Build history of the part. All positions in model axes, mm. Face numbers are marked on the shaded views. A direction names the side the tool comes from. Give positions to 0.01 mm unless a question says otherwise; leave off trailing zeros. Order: outer loops, then holes, each group sorted by start corner. A loop starts at its lowest first (then second) coordinate and runs counter-clockwise, first axis right, second up. Notation, with made-up numbers: (37.5, 67.5) - (44.5, 67.5) arc R30 ccw to (44.5, 104.5) - close; hole circle Ø2 at (66, 67.25). An arc over 180 degrees is marked (long way). Use a Markdown table: item, result. Add a question column.
(1) Slice it at C-C (z = -31). Write the cut outline in (x, y).
(2) Flat gauge pins, fed straight in: pin 1 (9.5 mm diameter, centred on x = 136, y = -14, fed in from -Z); pin 2 (11.5 mm diameter, centred on x = -51, y = -127, fed in from +Z); pin 3 (10 mm diameter, centred on y = -82, z = 22.5, fed in from +X). Where does each tip first touch, or does it go through?
(3) Slice it at A-A (x = 0). Count the separate pieces of the cut face and the enclosed holes in it, then the cut area to 3 significant figures.
(4) Wall check: line 1 (Y direction, x = 0, z = 38); line 2 (X direction, y = 94, z = 11); line 3 (X direction, y = 53, z = 17). Give the ranges that are in metal, low to high.
(5) Mould opens along Y. For the marked faces 3 and 4 say: +Y half, -Y half, draft (parallel to the pull), parting line (faces both ways), or undercut.
(6) Which spindle directions (+Z, -Z, +X, -X, +Y, -Y) get a long thin tool onto all of the face, cutting with end or side? Do the marked faces 1 and 2. Say none if no direction does.
from build123d import *

# Parameters (mm, degrees)
CUT_EXTRUDE1_DEPTH      = 246.560583156
CUT_EXTRUDE1_DEPTH_BACK = 246.560583156


with BuildPart() as part:
    # Sketch2 → Revolve1 (revolve)
    with BuildSketch(Plane(origin=(0, 0, 0), x_dir=(1, 0, 0), z_dir=(0, 1, 0))):
        with BuildLine():
            Line((-47.5, -40), (-114, -40))
            ThreePointArc((-114, -40), (-123.899494937, -35.899494937), (-128, -26))
            Line((-128, -26), (-130, -26))
            ThreePointArc((-130, -26), (-130.749756335, -18.015609771), (-131, -10))
            Line((-131, -10), (-151, -10))
            ThreePointArc((-151, -10), (-157.444175053, -16.906401533), (-160, -26))
            Line((-160, -26), (-170, -26))
            Line((-170, -26), (-170, -24))
            Line((-170, -24), (-164, -24))
            ThreePointArc((-164, -24), (-158.990908339, 0), (-164, 24))
            Line((-164, 24), (-170, 24))
            Line((-170, 24), (-170, 26))
            Line((-170, 26), (-160, 26))
            ThreePointArc((-160, 26), (-157.444175053, 16.906401533), (-151, 10))
            Line((-151, 10), (-131, 10))
            ThreePointArc((-131, 10), (-130.749756335, 18.015609771), (-130, 26))
            Line((-130, 26), (-128, 26))
            ThreePointArc((-128, 26), (-123.899494937, 35.899494937), (-114, 40))
            Line((-114, 40), (-47.5, 40))
            Line((-47.5, 40), (-47.5, 37))
            Line((-47.5, 37), (-30, 37))
            Line((-30, 37), (-30, -37))
            Line((-30, -37), (-47.5, -37))
            Line((-47.5, -37), (-47.5, -40))
        make_face()
    revolve(axis=Axis((0, 0, -135.367425902), (0, 0, 1)))

    # Sketch3 → Cut-Extrude1 (cut, two sides: drawn at the far end of the back side and taken through both)
    with BuildSketch(Plane.XY.offset(10).offset(-CUT_EXTRUDE1_DEPTH_BACK)):
        with BuildLine():
            ThreePointArc((-16.775359417, 141.517465908), (-17.663637735, 146.86526576), (-22.5, 149.314265896))
            ThreePointArc((-22.5, 149.314265896), (-65.516444607, 136.046299053), (-102.710073317, 110.687130414))
            ThreePointArc((-102.710073317, 110.687130414), (-103.810790461, 105.378983525), (-100.183544647, 101.350200901))
            Line((-100.183544647, 101.350200901), (-91.789558594, 98.103510563))
            ThreePointArc((-91.789558594, 98.103510563), (-89.333916802, 97.632512022), (-86.869399468, 98.054614557))
            ThreePointArc((-86.869399468, 98.054614557), (-56.838769824, 118.026921695), (-22.5, 129.053283569))
            ThreePointArc((-22.5, 129.053283569), (-20.633385525, 130.716944184), (-19.470559398, 132.930505034))
            Line((-19.470559398, 132.930505034), (-16.775359417, 141.517465908))
        make_face()
        with BuildLine():
            Line((-97.575757874, 87.406930362), (-113.234667829, 99.894494351))
            ThreePointArc((-113.234667829, 99.894494351), (-118.056553853, 94.146960081), (-122.587014857, 88.167022114))
            Line((-122.587014857, 88.167022114), (-106.928104902, 75.679458125))
            ThreePointArc((-106.928104902, 75.679458125), (-102.419924203, 81.677164043), (-97.575757874, 87.406930362))
        make_face()
        with BuildLine():
            ThreePointArc((-121.102075685, 75.119192657), (-125.836986444, 77.759007373), (-130.767114401, 75.504713703))
            ThreePointArc((-130.767114401, 75.504713703), (-147.214114739, 33.600661027), (-150.577366523, -11.289671876))
            ThreePointArc((-150.577366523, -11.289671876), (-147.113576085, -15.459822645), (-141.70219622, -15.135832553))
            Line((-141.70219622, -15.135832553), (-133.9302668, -10.597428308))
            ThreePointArc((-133.9302668, -10.597428308), (-132.030957698, -8.971193032), (-130.824369324, -6.781179166))
            ThreePointArc((-130.824369324, -6.781179166), (-127.715556496, 29.150242348), (-114.926440552, 62.872197846))
            ThreePointArc((-114.926440552, 62.872197846), (-115.063327708, 65.368851235), (-116.068949037, 67.658117926))
            Line((-116.068949037, 67.658117926), (-121.102075685, 75.119192657))
        make_face()
        with BuildLine():
            Line((-129.174979886, -21.790469739), (-148.701321217, -26.247229726))
            ThreePointArc((-148.701321217, -26.247229726), (-147.214114739, -33.600661027), (-145.363507208, -40.871148409))
            Line((-145.363507208, -40.871148409), (-125.837165877, -36.414388422))
            ThreePointArc((-125.837165877, -36.414388422), (-127.715556496, -29.150242348), (-129.174979886, -21.790469739))
        make_face()
        with BuildLine():
            ThreePointArc((-134.23645893, -47.845364818), (-139.252517754, -49.901369561), (-140.563924495, -55.161427924))
            ThreePointArc((-140.563924495, -55.161427924), (-118.056553853, -94.146960081), (-85.056831518, -124.765120976))
            ThreePointArc((-85.056831518, -124.765120976), (-79.636838347, -124.65706704), (-76.516203841, -120.224275379))
            Line((-76.516203841, -120.224275379), (-75.218752425, -111.318287515))
            ThreePointArc((-75.218752425, -111.318287515), (-75.305994506, -108.819406755), (-76.265920748, -106.510606666))
            ThreePointArc((-76.265920748, -106.510606666), (-102.419924203, -81.677164043), (-120.810927296, -50.652935214))
            ThreePointArc((-120.810927296, -50.652935214), (-122.848237262, -49.203319975), (-125.265052676, -48.562211955))
            Line((-125.265052676, -48.562211955), (-134.23645893, -47.845364818))
        make_face()
        with BuildLine():
            Line((-63.502807355, -114.579201682), (-72.192846774, -132.624254474))
            ThreePointArc((-72.192846774, -132.624254474), (-65.516444607, -136.046299053), (-58.678313755, -139.13251056))
            Line((-58.678313755, -139.13251056), (-49.988274336, -121.087457769))
            ThreePointArc((-49.988274336, -121.087457769), (-56.838769824, -118.026921695), (-63.502807355, -114.579201682))
        make_face()
        with BuildLine():
            ThreePointArc((-46.288050676, -134.781386717), (-47.808062962, -139.984997413), (-44.513232463, -144.289889236))
            ThreePointArc((-44.513232463, -144.289889236), (0, -151), (44.513232463, -144.289889236))
            ThreePointArc((44.513232463, -144.289889236), (47.808062962, -139.984997413), (46.288050676, -134.781386717))
            Line((46.288050676, -134.781386717), (40.134016708, -128.214205744))
            ThreePointArc((40.134016708, -128.214205744), (38.125918511, -126.724387679), (35.722321693, -126.035374927))
            ThreePointArc((35.722321693, -126.035374927), (0, -131), (-35.722321693, -126.035374927))
            ThreePointArc((-35.722321693, -126.035374927), (-38.125918511, -126.724387679), (-40.134016708, -128.214205744))
            Line((-40.134016708, -128.214205744), (-46.288050676, -134.781386717))
        make_face()
        with BuildLine():
            ThreePointArc((85.056831518, -124.765120976), (118.056553853, -94.146960081), (140.563924495, -55.161427924))
            ThreePointArc((140.563924495, -55.161427924), (139.252517754, -49.901369561), (134.23645893, -47.845364818))
            Line((134.23645893, -47.845364818), (125.265052676, -48.562211955))
            ThreePointArc((125.265052676, -48.562211955), (122.848237262, -49.203319975), (120.810927296, -50.652935214))
            ThreePointArc((120.810927296, -50.652935214), (102.419924203, -81.677164043), (76.265920748, -106.510606666))
            ThreePointArc((76.265920748, -106.510606666), (75.305994506, -108.819406755), (75.218752425, -111.318287515))
            Line((75.218752425, -111.318287515), (76.516203841, -120.224275379))
            ThreePointArc((76.516203841, -120.224275379), (79.636838347, -124.65706704), (85.056831518, -124.765120976))
        make_face()
        with BuildLine():
            ThreePointArc((145.363507208, -40.871148409), (147.214114739, -33.600661027), (148.701321217, -26.247229726))
            Line((148.701321217, -26.247229726), (129.174979886, -21.790469739))
            ThreePointArc((129.174979886, -21.790469739), (127.715556496, -29.150242348), (125.837165877, -36.414388422))
            Line((125.837165877, -36.414388422), (145.363507208, -40.871148409))
        make_face()
        with BuildLine():
            ThreePointArc((151, 0), (145.854095374, 39.084304557), (130.767114401, 75.504713703))
            ThreePointArc((130.767114401, 75.504713703), (125.836986444, 77.759007373), (121.102075685, 75.119192657))
            Line((121.102075685, 75.119192657), (116.068949037, 67.658117926))
            ThreePointArc((116.068949037, 67.658117926), (115.063327708, 65.368851235), (114.926440552, 62.872197846))
            ThreePointArc((114.926440552, 62.872197846), (126.918012339, 32.447159257), (131, 0))
            ThreePointArc((131, 0), (130.95608497, -3.391726589), (130.824369324, -6.781179166))
            ThreePointArc((130.824369324, -6.781179166), (132.030957698, -8.971193032), (133.9302668, -10.597428308))
            Line((133.9302668, -10.597428308), (141.70219622, -15.135832553))
            ThreePointArc((141.70219622, -15.135832553), (147.113576085, -15.459822645), (150.577366523, -11.289671876))
            ThreePointArc((150.577366523, -11.289671876), (150.894304639, -5.648789917), (151, 0))
        make_face()
        with BuildLine():
            ThreePointArc((122.587014857, 88.167022114), (118.056553853, 94.146960081), (113.234667829, 99.894494351))
            Line((113.234667829, 99.894494351), (97.575757874, 87.406930362))
            ThreePointArc((97.575757874, 87.406930362), (102.419924203, 81.677164043), (106.928104902, 75.679458125))
            Line((106.928104902, 75.679458125), (122.587014857, 88.167022114))
        make_face()
        with BuildLine():
            ThreePointArc((102.710073317, 110.687130414), (65.516444607, 136.046299053), (22.5, 149.314265896))
            ThreePointArc((22.5, 149.314265896), (17.663637735, 146.86526576), (16.775359417, 141.517465908))
            Line((16.775359417, 141.517465908), (19.470559398, 132.930505034))
            ThreePointArc((19.470559398, 132.930505034), (20.633385525, 130.716944184), (22.5, 129.053283569))
            ThreePointArc((22.5, 129.053283569), (56.838769824, 118.026921695), (86.869399468, 98.054614557))
            ThreePointArc((86.869399468, 98.054614557), (89.333916802, 97.632512022), (91.789558594, 98.103510563))
            Line((91.789558594, 98.103510563), (100.183544647, 101.350200901))
            ThreePointArc((100.183544647, 101.350200901), (103.810790461, 105.378983525), (102.710073317, 110.687130414))
        make_face()
        with BuildLine():
            ThreePointArc((7.5, 150.813626705), (0, 151), (-7.5, 150.813626705))
            Line((-7.5, 150.813626705), (-7.5, 130.785129124))
            ThreePointArc((-7.5, 130.785129124), (0, 131), (7.5, 130.785129124))
            Line((7.5, 130.785129124), (7.5, 150.813626705))
        make_face()
        with BuildLine():
            ThreePointArc((58.678313755, -139.13251056), (65.516444607, -136.046299053), (72.192846774, -132.624254474))
            Line((72.192846774, -132.624254474), (63.502807355, -114.579201682))
            ThreePointArc((63.502807355, -114.579201682), (56.838769824, -118.026921695), (49.988274336, -121.087457769))
            Line((49.988274336, -121.087457769), (58.678313755, -139.13251056))
        make_face()
    extrude(amount=CUT_EXTRUDE1_DEPTH + CUT_EXTRUDE1_DEPTH_BACK, mode=Mode.SUBTRACT)


solid = part.part
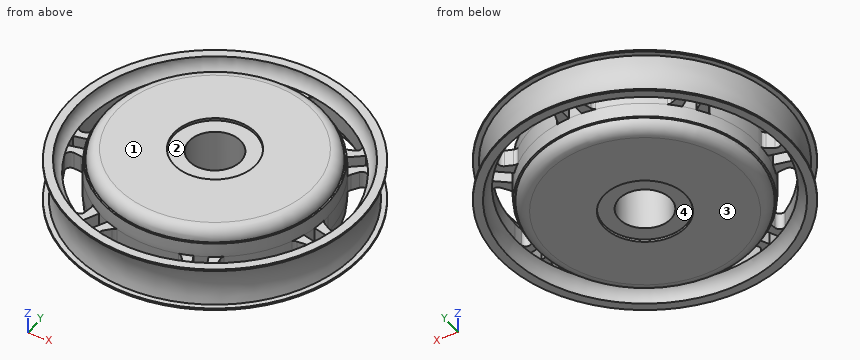
Solution:
| question | item | result |
|---|---|---|
| 1 | outline | circle Ø254.15 at (0, 0); hole circle Ø60 at (0, 0) |
| 2 | pin 1 | z = -10 |
| 2 | pin 2 | z = 10 |
| 2 | pin 3 | x = 151.44 |
| 3 | separate pieces | 4 |
| 3 | enclosed holes | 0 |
| 3 | area | 16,300 mm2 |
| 4 | line 1 | -121.21 to -47.5, 47.5 to 121.21 |
| 4 | line 2 | -129.49 to -119.94, -91.24 to 91.24, 119.94 to 129.49 |
| 4 | line 3 | -152.5 to -148.31, -119.59 to 119.59, 148.31 to 152.5 |
| 5 | face 3 | draft |
| 5 | face 4 | undercut |
| 6 | face 1 | +Z, +X, -X, +Y, -Y |
| 6 | face 2 | +Z |
